Check sheet for the modelled part. Datum: model origin and axes. Units: mm. Face numbers are marked on the shaded views. A direction names the side the tool comes from. Coordinates: 2 decimals unless noted, no trailing zeros. Order: outer loops, then holes, each group sorted by start corner. A loop starts at its lowest first (then second) coordinate and runs counter-clockwise, first axis right, second up.
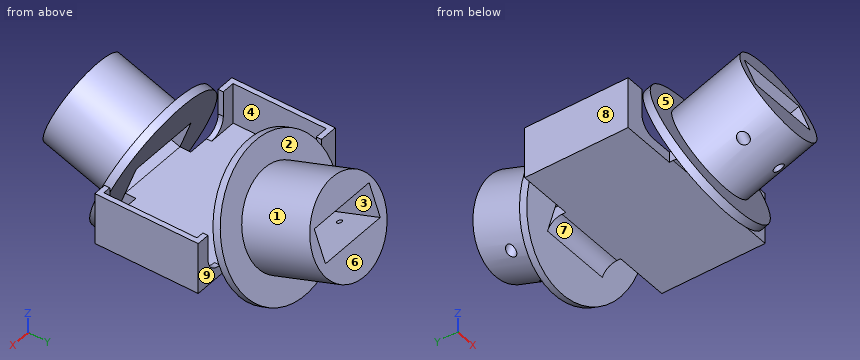
from build123d import *

# Parameters (mm, degrees)
BOX005_W               = 66
BOX005_H               = 36
BOX005_DEPTH           = 20
BOX006_W               = 58
BOX006_H               = 40
BOX006_DEPTH           = 20
BOX004_W               = 70
BOX004_H               = 40
BOX004_DEPTH           = 20
BOX002_W               = 28
BOX002_H               = 58
BOX002_DEPTH           = 4.1
BOX003_W               = 70
BOX003_H               = 40
BOX003_DEPTH           = 4.1
CYLINDER007_R          = 1
CYLINDER007_DEPTH      = 36
CYLINDER006_R          = 2
CYLINDER006_DEPTH      = 36
BOX_W                  = 16
BOX_H                  = 26
BOX_DEPTH              = 12
FILLET006_R            = 1
BOX001_W               = 28
BOX001_H               = 51
BOX001_DEPTH           = 12.6
CYLINDER005_R          = 18
CYLINDER005_DEPTH      = 31
CYLINDER005_ROLL_ANGLE = 90.0000000001
CYLINDER008_R          = 18
CYLINDER008_DEPTH      = 3
CYLINDER008_ROLL_ANGLE = 90.0000000001
CYLINDER009_R          = 28
CYLINDER009_DEPTH      = 3
CYLINDER009_ROLL_ANGLE = 90.0000000001
FUSION005_ROLL_ANGLE   = -20
FILLET_R               = 6
FILLET008_R            = 6


with BuildPart() as cubo005:
    # Box005 → Box005 (new body)
    with BuildSketch(Plane(origin=(-33, 27, -17), x_dir=(1, 0, 0), z_dir=(0, 0, 1))):
        with Locations((33, 18)):
            Rectangle(BOX005_W, BOX005_H)
    extrude(amount=BOX005_DEPTH)


with BuildPart() as fusion006:
    # Box006 → Box006 (new body)
    with BuildSketch(Plane(origin=(-28, 25, -17), x_dir=(1, 0, 0), z_dir=(0, 0, 1))):
        with Locations((29, 20)):
            Rectangle(BOX006_W, BOX006_H)
    extrude(amount=BOX006_DEPTH)

    # Fusion006: union Cubo005
    add(cubo005.part)


with BuildPart() as cut009:
    # Box004 → Box004 (new body)
    with BuildSketch(Plane(origin=(-35, 25, -17), x_dir=(1, 0, 0), z_dir=(0, 0, 1))):
        with Locations((35, 20)):
            Rectangle(BOX004_W, BOX004_H)
    extrude(amount=BOX004_DEPTH)

    # Cut009: cut Fusion006
    add(fusion006.part, mode=Mode.SUBTRACT)


with BuildPart() as cubo002:
    # Box002 → Box002 (new body)
    with BuildSketch(Plane(origin=(-14, 16, -17), x_dir=(1, 0, 0), z_dir=(0, 0, 1))):
        with Locations((14, 29)):
            Rectangle(BOX002_W, BOX002_H)
    extrude(amount=BOX002_DEPTH)


with BuildPart() as fusion007:
    # Box003 → Box003 (new body)
    with BuildSketch(Plane(origin=(-35, 25, -17), x_dir=(1, 0, 0), z_dir=(0, 0, 1))):
        with Locations((35, 20)):
            Rectangle(BOX003_W, BOX003_H)
    extrude(amount=BOX003_DEPTH)

    # Fusion007: union Cut009, Cubo002
    add(cut009.part)
    add(cubo002.part)


with BuildPart() as cilindro007:
    # Cylinder007 → Cylinder007 (new body)
    with BuildSketch(Plane(origin=(9, 5.75, -40), x_dir=(1, 0, 0), z_dir=(0, 0, 1))):
        Circle(CYLINDER007_R)
    extrude(amount=CYLINDER007_DEPTH)


with BuildPart() as fusion003:
    # Cylinder006 → Cylinder006 (new body)
    with BuildSketch(Plane(origin=(9, 5.75, -45), x_dir=(1, 0, 0), z_dir=(0, 0, 1))):
        Circle(CYLINDER006_R)
    extrude(amount=CYLINDER006_DEPTH)

    # Fusion003: union Cilindro007
    add(cilindro007.part)


with BuildPart() as fusion004:
    # Part__Mirroring: instance of Fusion003
    add(fusion003.part.mirror(Plane(origin=(0, 0, 0), x_dir=(0, -1, 0), z_dir=(1, 0, 0))))

    # Fusion004: union Fusion003
    add(fusion003.part)


with BuildPart() as fillet006:
    # Box → Box (new body)
    with BuildSketch(Plane(origin=(-8, -8, -5), x_dir=(1, 0, 0), z_dir=(0, 0, 1))):
        with Locations((8, 13)):
            Rectangle(BOX_W, BOX_H)
    extrude(amount=BOX_DEPTH)

    # Fillet006
    fillet006_edges = [fillet006.edges().sort_by_distance(p)[0] for p in [
        (-8, 5, 7),
        (8, 5, 7),
    ]]
    fillet(fillet006_edges, radius=FILLET006_R)


with BuildPart() as fusion002:
    # Box001 → Box001 (new body)
    with BuildSketch(Plane(origin=(-14, -12, -5), x_dir=(1, 0, 0), z_dir=(0, 0, 1))):
        with Locations((14, 25.5)):
            Rectangle(BOX001_W, BOX001_H)
    extrude(amount=BOX001_DEPTH)

    # Fusion002: union Fillet006
    add(fillet006.part)


with BuildPart() as cut004:
    # Cylinder005 → Cylinder005 (new body)
    with BuildSketch(Plane.XY):
        Circle(CYLINDER005_R)
    extrude(amount=CYLINDER005_DEPTH)


with BuildPart() as cut004_1:
    # Cylinder005 roll: moved
    add(cut004.part.rotate(Axis((0, 0, 0), (1, 0, 0)), CYLINDER005_ROLL_ANGLE))


with BuildPart() as cut004_2:
    # Cylinder005 placement: moved
    add(cut004_1.part.moved(Location((0, 24, 0))))

    # Cut003: cut Fusion002
    add(fusion002.part, mode=Mode.SUBTRACT)

    # Cut004: cut Fusion004
    add(fusion004.part, mode=Mode.SUBTRACT)


with BuildPart() as cilindro008:
    # Cylinder008 → Cylinder008 (new body)
    with BuildSketch(Plane.XY):
        Circle(CYLINDER008_R)
    extrude(amount=CYLINDER008_DEPTH)


with BuildPart() as cilindro008_1:
    # Cylinder008 roll: moved
    add(cilindro008.part.rotate(Axis((0, 0, 0), (1, 0, 0)), CYLINDER008_ROLL_ANGLE))


with BuildPart() as cilindro008_2:
    # Cylinder008 placement: moved
    add(cilindro008_1.part.moved(Location((0, 24, 0))))


with BuildPart() as fusion005:
    # Cylinder009 → Cylinder009 (new body)
    with BuildSketch(Plane.XY):
        Circle(CYLINDER009_R)
    extrude(amount=CYLINDER009_DEPTH)


with BuildPart() as fusion005_1:
    # Cylinder009 roll: moved
    add(fusion005.part.rotate(Axis((0, 0, 0), (1, 0, 0)), CYLINDER009_ROLL_ANGLE))


with BuildPart() as fusion005_2:
    # Cylinder009 placement: moved
    add(fusion005_1.part.moved(Location((0, 24, 0))))

    # Cut005: cut Cilindro008
    add(cilindro008_2.part, mode=Mode.SUBTRACT)

    # Fusion005: union Cut004
    add(cut004_2.part)


with BuildPart() as fusion005_3:
    # Fusion005 roll: moved
    add(fusion005_2.part.rotate(Axis((0, 0, 0), (1, 0, 0)), FUSION005_ROLL_ANGLE))


with BuildPart() as fusion005_4:
    # Fusion005 placement: moved
    add(fusion005_3.part)


with BuildPart() as part_mirroring004:
    # Part__Mirroring004: instance of Fusion005
    add(fusion005_4.part.mirror(Plane(origin=(0, 45, 0), x_dir=(1, 0, 0), z_dir=(0, 1, 0))))


with BuildPart() as fillet008:
    # Fusion008 base: copy of Fusion005
    add(fusion005_4.part)

    # Fusion008: union Fusion007, Part__Mirroring004
    add(fusion007.part)
    add(part_mirroring004.part)

    # Fillet
    fillet_edges = [fillet008.edges().sort_by_distance(p)[0] for p in [
        (0, 19.352773, -17),
        (0, 70.647227, -17),
    ]]
    fillet(fillet_edges, radius=FILLET_R)

    # Fillet008
    fillet008_edges = [fillet008.edges().sort_by_distance(p)[0] for p in [
        (-28, 26, -12.9),
        (-28, 64, -12.9),
        (30, 64, -12.9),
        (30, 26, -12.9),
    ]]
    fillet(fillet008_edges, radius=FILLET008_R)


solid = fillet008.part
(1) Thickness scan on probe 1 along X at (y, z) = (60, 1.5); probe 2 along Z at (x, y) = (11.5, 40); probe 3 along X at (y, z) = (26, 0). Record the ranges inside material, lowest first.
Filled in:
probe 1: x = -35 to -33, 33 to 35
probe 2: z = -17 to -12.9
probe 3: x = -35 to -28, 30 to 35
(2) Go/stop test with flat-tipped pins: P1, Ø16, axis at x = -28, z = -3, coming from the -Y side; P2, Ø2, axis at y = 70, z = -16.5, coming from the +X side; P3, Ø24, axis at x = 6.5, y = 34, coming from the +Z side; P4, Ø6, axis at y = 45, z = -19.5, coming from the -X side. Record where each tip stops, or that it passes through.
Filled in:
P1: stops at y = 18.35
P2: stops at x = 26.9
P3: stops at z = 19.13
P4: stops at x = -35
(3) Cross-section at D-D (x = 26). Enter the section's corners in (y, z).
Filled in:
outline: (16.18, -16.95) - (19, -17.97) - (26.11, 1.56) - (23.29, 2.58) - close; (25, -17) - (65, -17) - (65, -12.56) - (63, -12.56) - (63, -12.9) - (27, -12.9) - (27, -12.56) - (25, -12.56) - close; (63.89, 1.56) - (71, -17.97) - (73.82, -16.95) - (66.71, 2.58) - close
(4) Cross-section at B-B (y = 50.5). Enter the section's corners in (x, z), and give its area (3 significant figures).
Filled in:
outline: (-35, -17) - (35, -17) - (35, 3) - (33, 3) - (33, -12.9) - (-33, -12.9) - (-33, 3) - (-35, 3) - close
area: 351 mm2
(5) Cross-section at A-A (x = -25). Enter the section's corners in (y, z).
Filled in:
outline: (15.42, -19.03) - (18.24, -20.06) - (26.87, 3.64) - (24.05, 4.67) - close; (25, -17) - (65, -17) - (65, -12.1) - (63, -12.1) - (63, -12.9) - (27, -12.9) - (27, -12.1) - (25, -12.1) - close; (63.13, 3.64) - (71.76, -20.06) - (74.58, -19.03) - (65.95, 4.67) - close
(6) Tool access check on the marked faces 5, 6, 7, 8 and 9. Record the directions out of +Z, -Z, +X, -X, +Y, -Y that give a thin tool (end or side, any length) a straight path to the whole face; none if there is none.
Filled in:
face 5: none
face 6: +Z, +X, -X, +Y
face 7: -Z, +X, -X
face 8: +Z, -Z, -X, +Y, -Y
face 9: -Z, +X
(7) Release check for a two-part mould opening along X. For the marked faces 1, 2, 3 and 4 record: +X half, -X half, draft (parallel to the pull), parting line (faces both ways), or undercut.
Filled in:
face 1: parting line
face 2: draft
face 3: undercut
face 4: undercut
(8) Cross-section at C-C (z = 15). Count the separate pieces of the cut face and the enclosed holes in it, and give its area (3 significant figures).
Filled in:
separate pieces: 4
enclosed holes: 0
area: 622 mm2
